Verification items for the finished model (mm, model axes). A direction names the side the tool comes from. Coordinates: 2 decimals unless noted, no trailing zeros. Loops run counter-clockwise (first coordinate to the right, second up) from the corner with the lowest first, then second, coordinate; pieces in that order, holes last. Notation, with made-up numbers: (5, 13.5) -> (31, 13.5) arc R19 ccw to (31, 29.5) -> close; hole circle Ø11 at (54, -28). An arc over 180 degrees is marked (long way). Use CSV: the item, a comma, the result in double quotes. Start each with the question number.
```python
from build123d import *

# Parameters (mm, degrees)
F1_DEPTH = 31.5
F2_DEPTH = 29
F3_DEPTH = 24
F5_DEPTH = 7.5


with BuildPart() as f1:
    # F0 (on Right) → F1 (new body, symmetric)
    with BuildSketch(Plane.YZ):
        Polygon((20.983844617, 45), (0, 0), (2.7584447974, 0), (23.7422894144, 45), align=None)
        Polygon((23.7422894144, 45), (2.7584447974, 0), (17.2415552026, 0), (38.2253998196, 45), align=None)
        Polygon((38.2253998196, 45), (17.2415552026, 0), (20, 0), (40.983844617, 45), align=None)
    extrude(amount=F1_DEPTH, both=True)

    # F0 (on Right) → F2 (cut, symmetric)
    with BuildSketch(Plane.YZ):
        Polygon((23.7422894144, 45), (2.7584447974, 0), (17.2415552026, 0), (38.2253998196, 45), align=None)
    extrude(amount=F2_DEPTH, both=True, mode=Mode.SUBTRACT)

    # F0 (on Right) → F3 (cut, symmetric)
    with BuildSketch(Plane.YZ):
        Polygon((20.983844617, 45), (0, 0), (2.7584447974, 0), (23.7422894144, 45), align=None)
        Polygon((23.7422894144, 45), (2.7584447974, 0), (17.2415552026, 0), (38.2253998196, 45), align=None)
        Polygon((38.2253998196, 45), (17.2415552026, 0), (20, 0), (40.983844617, 45), align=None)
    extrude(amount=F3_DEPTH, both=True, mode=Mode.SUBTRACT)

    # F4 (on Top) → F5 (join)
    with BuildSketch(Plane.XY):
        Polygon((-31.5, 50), (-31.5, 20), (-31.5, 0), (-31.5, -30), (-24, -22.5), (-24, 0), (-15.75, 0), (-8.25, 0), (8.25, 0), (15.75, 0), (24, 0), (24, -22.5), (31.5, -30), (31.5, 0), (31.5, 20), (31.5, 50), (24, 42.5), (24, 20), (15.75, 20), (8.25, 20), (-8.25, 20), (-15.75, 20), (-24, 20), (-24, 42.5), align=None)
        Polygon((-15.75, 34.25), (-15.75, 20), (-8.25, 20), (-8.25, 26.75), align=None)
        Polygon((-8.25, 0), (-15.75, 0), (-15.75, -14.25), (-8.25, -6.75), align=None)
        Polygon((15.75, 0), (8.25, 0), (8.25, -6.75), (15.75, -14.25), align=None)
        Polygon((8.25, 26.75), (8.25, 20), (15.75, 20), (15.75, 34.25), align=None)
    extrude(amount=-F5_DEPTH)


solid = f1.part
```
1. Release check for a two-part mould opening along X. For faces 1 (the flat face through (-24, 31, -4)), 2 (the flat face through (-28, 32, 0)), 3 (the flat face through (0, 0, -4)), 4 (the flat face through (-31.5, 16, 13)) record: released by +X, released by -X, zero draft, split by the parting line, or undercut.
2. Cross-section at D-D, the plane y = -25. Record the boundary of the cut face in (x, z), plus the area to 3 significant figures.
3. Set-up check for faces 5 (the flat face through (0, 10, 0)), 6 (the flat face through (11.9, -10.4, -3.7)), 7 (the flat face through (-24, 12, 23)), 8 (the flat face through (-8.25, 23, -4)): record each of +Z, -Z, +X, -X, +Y, -Y from which the full face is reachable in a straight line by a thin tool's end or side.
4. Cross-section at A-A, the plane y = -16.5. Record the boundary of the cut face in (x, z), plus the area to 4 significant figures.
5. Cross-section at C-C, the plane x = 26.5. Record the boundary of the cut face in (y, z).
6. Depth check by flat-ended pin: pin 1 (19 mm diameter, centred on y = 31, z = 22, fed in from -X); pin 2 (6 mm diameter, centred on x = 1, z = -5.5, fed in from +Y); pin 3 (2 mm diameter, centred on x = -26, y = 29, fed in from +Z); pin 4 (8 mm diameter, centred on x = 26.5, y = -13.5, fed in from +Z). Enter the tip coordinate at first touch or a pass-through.
7. Cross-section at B-B, the plane z = 18. Record the boundary of the cut face in (x, y).
8. Scan lines: line 1 (X direction, y = 23.5, z = -4); line 2 (X direction, y = 34.5, z = 36.5); line 3 (Z direction, x = 1, y = 1). Record each from-to range of solid material in increasing order.
Solution:
1,face 1,"undercut"
1,face 2,"zero draft"
1,face 3,"undercut"
1,face 4,"released by -X"
2,outline,"(-31.5, -7.5) -> (-26.5, -7.5) -> (-26.5, 0) -> (-31.5, 0) -> close; (26.5, -7.5) -> (31.5, -7.5) -> (31.5, 0) -> (26.5, 0) -> close"
2,area,"75.0 mm2"
3,face 5,"none"
3,face 6,"+Z, -Z, -Y"
3,face 7,"+Z, +Y, -Y"
3,face 8,"+Z, -Z, +Y"
4,outline,"(-31.5, -7.5) -> (-24, -7.5) -> (-24, 0) -> (-31.5, 0) -> close; (24, -7.5) -> (31.5, -7.5) -> (31.5, 0) -> (24, 0) -> close"
4,area,"112.5 mm2"
5,outline,"(-25, -7.5) -> (45, -7.5) -> (45, 0) -> (20, 0) -> (40.98, 45) -> (38.23, 45) -> (17.24, 0) -> (2.76, 0) -> (23.74, 45) -> (20.98, 45) -> (0, 0) -> (-25, 0) -> close"
6,pin 1,"stops at x = -31.5"
6,pin 2,"stops at y = 20"
6,pin 3,"stops at z = 27.36"
6,pin 4,"stops at z = 0"
7,outline,"(-31.5, 8.39) -> (-24, 8.39) -> (-24, 11.15) -> (-29, 11.15) -> (-29, 25.64) -> (-24, 25.64) -> (-24, 28.39) -> (-31.5, 28.39) -> close; (24, 8.39) -> (31.5, 8.39) -> (31.5, 28.39) -> (24, 28.39) -> (24, 25.64) -> (29, 25.64) -> (29, 11.15) -> (24, 11.15) -> close"
8,line 1,"x = -31.5 to -24, -15.75 to -8.25, 8.25 to 15.75, 24 to 31.5"
8,line 2,"x = -31.5 to -24, 24 to 31.5"
8,line 3,"z = -7.5 to 0"
